from build123d import *

# Parameters (mm, degrees)
SKETCH_2_R          = 30
EXTRUDE_1_DEPTH     = 3
SKETCH_3_R          = 3.5
CUT_EXTRUDE_1_DEPTH = 3
SKETCH_4_W          = 3
SKETCH_4_H          = 10
EXTRUDE_2_DEPTH     = 50
EXTRUDE_3_DEPTH     = 3
SKETCH_7_R          = 2
CUT_EXTRUDE_2_DEPTH = 3


with BuildPart() as part:
    # 草图2 → 凸台-拉伸1 (new body)
    with BuildSketch(Plane.XY):
        Circle(SKETCH_2_R)
    extrude(amount=EXTRUDE_1_DEPTH)

    # 草图3 → 切除-拉伸1 (cut)
    with BuildSketch(Plane.XY.offset(3)):
        with Locations((-17.67766953, 17.67766953)):
            Circle(SKETCH_3_R)
        with Locations(Location((17.67766953, 17.67766953, 0), (0, 0, 180))):
            Circle(SKETCH_3_R)
        with Locations((17.67766953, -17.67766953)):
            Circle(SKETCH_3_R)
        with Locations(Location((-17.67766953, -17.67766953, 0), (0, 0, 180))):
            Circle(SKETCH_3_R)
    extrude(amount=-CUT_EXTRUDE_1_DEPTH, mode=Mode.SUBTRACT)

    # 草图4 → 凸台-拉伸2 (add)
    with BuildSketch(Plane(origin=(0, 0, 0), x_dir=(0, 0, -1), z_dir=(1, 0, 0))):
        with Locations((-1.5, 0)):
            Rectangle(SKETCH_4_W, SKETCH_4_H)
    extrude(amount=EXTRUDE_2_DEPTH)

    # 草图5 → 凸台-拉伸3 (add)
    with BuildSketch(Plane.XY.offset(3)):
        with BuildLine():
            Line((57.5, 10), (57.5, -10))
            ThreePointArc((57.5, -10), (50, -17.5), (42.5, -10))
            Line((42.5, -10), (42.5, 10))
            ThreePointArc((42.5, 10), (50, 17.5), (57.5, 10))
        make_face()
    extrude(amount=-EXTRUDE_3_DEPTH)

    # 草图7 → 切除-拉伸2 (cut)
    with BuildSketch(Plane.XY.offset(3)):
        with Locations((50, 10)):
            Circle(SKETCH_7_R)
        with Locations((50, -10)):
            Circle(SKETCH_7_R)
    extrude(amount=-CUT_EXTRUDE_2_DEPTH, mode=Mode.SUBTRACT)


solid = part.part
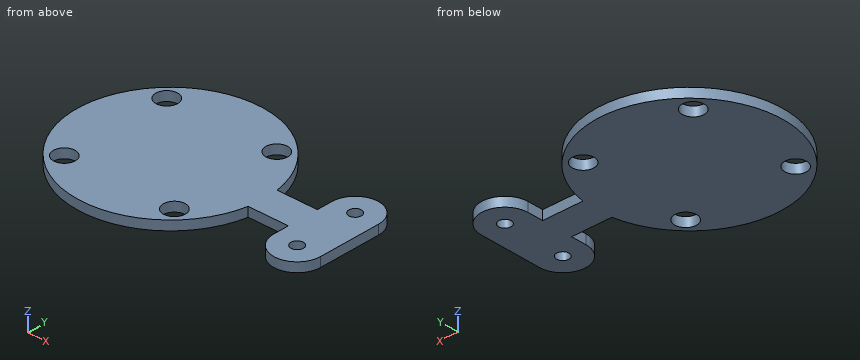
Design review of the part built by this model. Coordinates are the model's own, in mm. Round coordinates to 2 decimals unless told otherwise and drop trailing zeros. Write each loop counter-clockwise with the first axis right and the second up, starting at its lowest first coordinate (ties: lowest second). Pieces come first, ordered by that corner, then holes. Notation, with made-up numbers: (12.5, -20) - (45.5, -20) arc R13 ccw to (45.5, -8) - close; hole circle Ø11 at (69, -33.75). An arc over 180 degrees is marked (long way). Use a Markdown table: item, result. Add a question column.
1. We need section C-C (y = 6.5). State the section outline as (x, z) points, then the cut area to 3 significant figures.
2. We need section A-A (x = 50). State the section outline as (y, z) points, then the cut area to 3 significant figures.
3. Clearance check with flat-ended pins moving along their axes: pin 1 (3.5 mm diameter, centred on x = 50, y = -10, fed in from +Z); pin 2 (0.9 mm diameter, centred on x = 34.5, z = 2, fed in from -Y); pin 3 (0.9 mm diameter, centred on x = 35, z = 1.5, fed in from +Y); pin 4 (1.5 mm diameter, centred on x = 25.5, z = 0.5, fed in from +Y). State where each tip first meets the part, or that it passes through.
4. Wall thickness on probe 1 along Y at (x, z) = (17, 2.2); probe 2 along Y at (x, z) = (-20, 2.9); probe 3 along X at (y, z) = (-18, 2.35): over which ranges is each line inside the solid? List them lowest first.
5. We need section B-B (z = 0.5). State the section outline as (x, y) points.
Output:
| question | item | result |
|---|---|---|
| 1 | outline | (-29.29, 0) - (29.29, 0) - (29.29, 3) - (-29.29, 3) - close; (42.5, 0) - (57.5, 0) - (57.5, 3) - (42.5, 3) - close |
| 1 | area | 221 mm2 |
| 2 | outline | (-17.5, 0) - (-12, 0) - (-12, 3) - (-17.5, 3) - close; (-8, 0) - (8, 0) - (8, 3) - (-8, 3) - close; (12, 0) - (17.5, 0) - (17.5, 3) - (12, 3) - close |
| 2 | area | 81.0 mm2 |
| 3 | pin 1 | passes through |
| 3 | pin 2 | stops at y = -5 |
| 3 | pin 3 | stops at y = 5 |
| 3 | pin 4 | stops at y = 16.95 |
| 4 | probe 1 | y = -24.72 to -21.11, -14.24 to 14.24, 21.11 to 24.72 |
| 4 | probe 2 | y = -22.36 to -20.3, -15.06 to 15.06, 20.3 to 22.36 |
| 4 | probe 3 | x = -24 to -21.16, -14.19 to 14.19, 21.16 to 24 |
| 5 | outline | (29.58, -5) - (42.5, -5) - (42.5, -10) arc R7.5 ccw to (57.5, -10) - (57.5, 10) arc R7.5 ccw to (42.5, 10) - (42.5, 5) - (29.58, 5) arc R30 ccw (long way) to start; hole circle Ø7 at (-17.68, -17.68); hole circle Ø7 at (-17.68, 17.68); hole circle Ø7 at (17.68, -17.68); hole circle Ø7 at (17.68, 17.68); hole circle Ø4 at (50, -10); hole circle Ø4 at (50, 10) |
